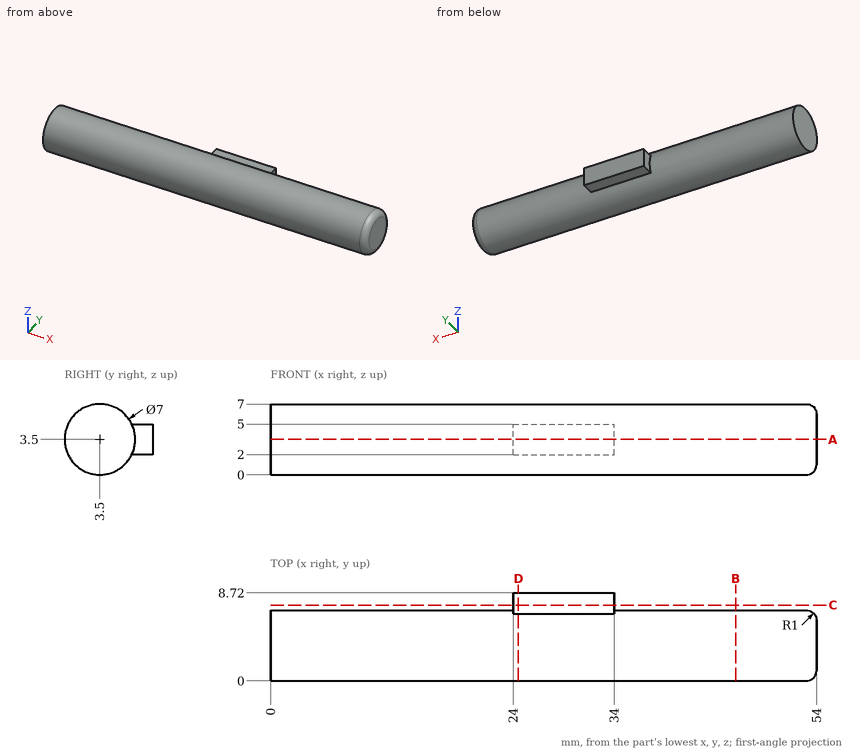
Input: dimensioned drawing with shaded views. Units: mm. Origin: part minimum x, y, z. Coordinates: 2 decimals unless noted, no trailing zeros. Loops run counter-clockwise (first coordinate to the right, second up) from the corner with the lowest first, then second, coordinate; pieces in that order, holes last. Notation, with made-up numbers: M 46.25,-27 L 92.25,-27 A23 cw 92.25,-15 Z; hole C 51,41 d7. An arc over 180 degrees is marked long. One line per item, written item: value.
(1) Line query: line 1 along Y through (x, z) = (19.5, 3.75); line 2 along Z through (x, y) = (31.5, 6.75). Output: solid intervals per line, ascending. Write a range as from..to.
Filled in:
line 1: 0.01..6.99
line 2: 2..5
(2) Section D-D (x = 24.5). Output: boundary loops of the cut face in (y, z).
Filled in:
outline: M 6.66,2 L 8.72,2 L 8.72,5 L 6.66,5 A3.5 ccw long Z
(3) Pin query (flat end, axial travel): pin 1 (0.6 mm diameter, centred on x = 27.5, y = 7.5, fed in from +Z); pin 2 (1 mm diameter, centred on x = 28, y = 7.5, fed in from -Z); pin 3 (1 mm diameter, centred on y = 7.5, z = 4, fed in from -X). Return the tip coordinate at first contact, or that it passes through.
Filled in:
pin 1: z = 5
pin 2: z = 2
pin 3: x = 24
(4) Section A-A (z = 3.5). Output: boundary loops of the cut face in (x, y).
Filled in:
outline: M 0,0 L 53,0 A1 ccw 54,1 L 54,6 A1 ccw 53,7 L 34,7 L 34,8.72 L 24,8.72 L 24,7 L 0,7 Z
(5) Section C-C (y = 7.5). Output: boundary loops of the cut face in (x, z).
Filled in:
outline: M 24,2 L 34,2 L 34,5 L 24,5 Z
(6) Section B-B (x = 46). Output: boundary loops of the cut face in (y, z), and give its area (3 significant figures).
Filled in:
outline: C 3.5,3.5 d7
area: 38.5 mm^2
